Build history of the part. All positions in model axes, mm. Face numbers are marked on the shaded views. A direction names the side the tool comes from. Round coordinates to 2 decimals unless told otherwise and drop trailing zeros. Order: outer loops, then holes, each group sorted by start corner. A loop starts at its lowest first (then second) coordinate and runs counter-clockwise, first axis right, second up. Notation, with made-up numbers: M 75,86.25 L 108,86.25 A33 ccw 108,123.25 Z; hole C 46,34.5 d8. An arc over 180 degrees is marked long. One line per item, written item: value. Start each with the question number.
Item 1: Band-saw the part on B-B, the plane z = -50. Write the cut outline in (x, y).
Item 2: Probe L1, parallel to Y at x = 2.05, z = -10; L2, parallel to Y at x = 3.35, z = 0; L3, parallel to Z at x = 2.3, y = 0. List the from-to ranges inside material, lowest first.
Item 3: Pin check, flat tips, straight feed: pin 1 (1.5 mm diameter, centred on x = 10, y = 26, fed in from -Z); pin 2 (6 mm diameter, centred on y = 40.5, z = 0.5, fed in from -X); pin 3 (12 mm diameter, centred on x = 10.5, y = 39, fed in from -Z); pin 4 (2.5 mm diameter, centred on x = 2.5, z = -32.5, fed in from +Y). Stop position of each tip, or through.
Item 4: Band-saw the part on D-D, the plane z = -10. Write the cut outline in (x, y).
Item 5: Band-saw the part on A-A, the plane y = 0. Write the cut outline in (x, z), then the cut area to 3 significant figures.
Item 6: Tool access for the marked faces 4, 5, 6 and 7: list every direction of +Z, -Z, +X, -X, +Y, -Y with a clear straight run to the whole face (end or side of a thin tool).
Item 7: Two-plate mould, pull along Y, no slides. Class the marked faces 1, 2 and 3: +Y half, -Y half, draft (parallel to the pull), parting line (faces both ways), or undercut.
Item 8: Band-saw the part on C-C, the plane x = 12.5. Write the cut outline in (y, z), then the cut area to 3 significant figures.
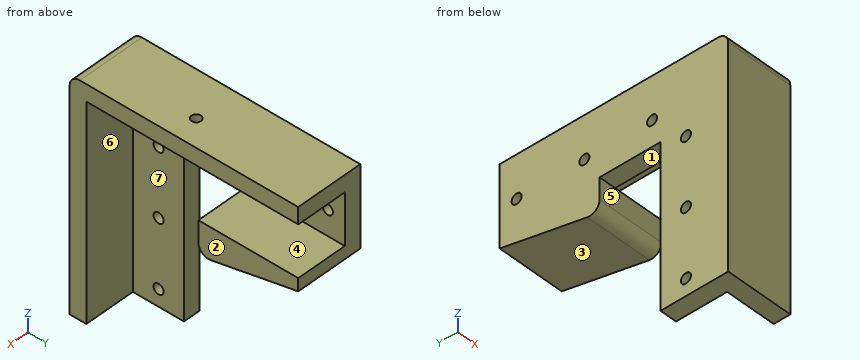
```python
from build123d import *

# Parameters (mm, degrees)
SKETCH_1_R          = 1.5
EXTRUDE_1_DEPTH     = 20
CUT_EXTRUDE_1_DEPTH = 15
SKETCH_3_R          = 1.4
CUT_EXTRUDE_2_DEPTH = 86.695740851
FILLET_1_R          = 3


with BuildPart() as part:
    # 草图1 → 凸台-拉伸1 (new body)
    with BuildSketch(Plane(origin=(0, 0, 0), x_dir=(0, 0, -1), z_dir=(1, 0, 0))):
        Polygon((-12.5, -12.5), (55, -12.5), (55, 7.5), (7.5, 7.5), (7.5, 25.5), (17.5, 25.5), (11.229581431, 55), (-12.5, 55), align=None)
        with Locations((0, 10)):
            Circle(SKETCH_1_R, mode=Mode.SUBTRACT)
        with Locations((0, 30)):
            Circle(SKETCH_1_R, mode=Mode.SUBTRACT)
        with Locations((10, 0)):
            Circle(SKETCH_1_R, mode=Mode.SUBTRACT)
        with Locations((30, 0)):
            Circle(SKETCH_1_R, mode=Mode.SUBTRACT)
        with Locations((50, 0)):
            Circle(SKETCH_1_R, mode=Mode.SUBTRACT)
        with Locations((0, 50)):
            Circle(SKETCH_1_R, mode=Mode.SUBTRACT)
    extrude(amount=EXTRUDE_1_DEPTH)

    # 草图2 → 切除-拉伸1 (cut)
    with BuildSketch(Plane.ZY.offset(-20)):
        Polygon((7.6, 55), (7.6, -7.6), (-55, -7.6), (-55, 7.5), (-7.5, 7.5), (-7.5, 55), align=None)
    extrude(amount=CUT_EXTRUDE_1_DEPTH, mode=Mode.SUBTRACT)

    # 草图3 → 切除-拉伸2 (cut, through all)
    with BuildSketch(Plane(origin=(0, 0, 7.6), x_dir=(-1, 0, 0), z_dir=(0, 0, -1))):
        with Locations(Location((-12.5, 18, 0), (0, 0, 90))):
            Circle(SKETCH_3_R)
    extrude(amount=-CUT_EXTRUDE_2_DEPTH, mode=Mode.SUBTRACT)

    # 圆角1
    fillet_1_edges = [part.edges().sort_by_distance(p)[0] for p in [
        (10, -12.5, 12.5),
        (10, 25.5, -17.5),
    ]]
    fillet(fillet_1_edges, radius=FILLET_1_R)


solid = part.part
```
Output:
1. outline: M 0,-12.5 L 20,-12.5 L 20,-7.6 L 5,-7.6 L 5,-1.5 L 0,-1.5 Z; M 0,1.5 L 5,1.5 L 5,7.5 L 0,7.5 Z
2. L1: y = -12.5 to -1.5, 1.5 to 7.5, 25.5 to 55
2. L2: y = -12.5 to 8.5, 11.5 to 28.5, 31.5 to 48.5, 51.5 to 55
2. L3: z = -55 to -51.5, -48.5 to -31.5, -28.5 to -11.5, -8.5 to 12.5
3. pin 1: stops at z = -16.23
3. pin 2: stops at x = 0
3. pin 3: stops at z = -15.91
3. pin 4: stops at y = 7.5
4. outline: M 0,-12.5 L 20,-12.5 L 20,-7.6 L 5,-7.6 L 5,-1.5 L 0,-1.5 Z; M 0,1.5 L 5,1.5 L 5,7.5 L 0,7.5 Z; M 0,25.5 L 20,25.5 L 20,55 L 0,55 Z
5. outline: M 0,-55 L 5,-55 L 5,-51.5 L 0,-51.5 Z; M 0,-48.5 L 5,-48.5 L 5,-31.5 L 0,-31.5 Z; M 0,-28.5 L 5,-28.5 L 5,-11.5 L 0,-11.5 Z; M 0,-8.5 L 5,-8.5 L 5,7.6 L 20,7.6 L 20,12.5 L 0,12.5 Z
5. area: 366 mm²
6. face 4: +X, +Y
6. face 5: -Z, +X, -X
6. face 6: -Z, +X
6. face 7: +X
7. face 1: undercut
7. face 2: draft
7. face 3: +Y half
8. outline: M -12.5,-55 L -7.6,-55 L -7.6,7.6 L 16.6,7.6 L 16.6,12.5 L -9.5,12.5 A3 ccw -12.5,9.5 Z; M 19.4,7.6 L 55,7.6 L 55,12.5 L 19.4,12.5 Z; M 25.5,-13.8 A3 ccw 29.12,-16.73 L 55,-11.23 L 55,-7.5 L 25.5,-7.5 Z
8. area: 821 mm²
